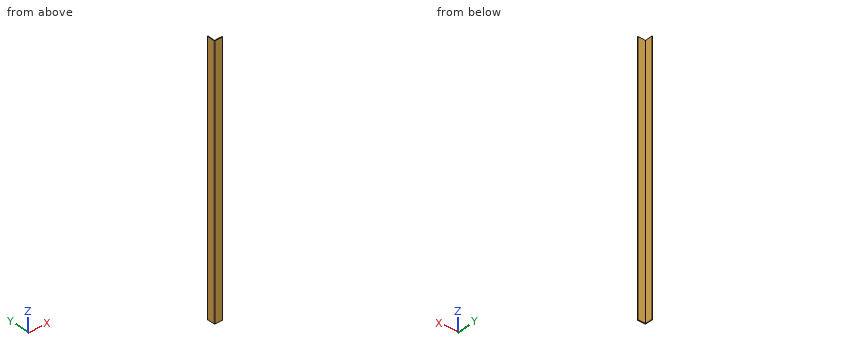
Autodesk Inventor part; units mm, degrees
ref_plane "Work Plane2" through (0, 30, 0) normal (-0.7071, 0.7071, 0) x (0, 0, -1)
ref_plane "Work Plane4" through (15.0001, 14.9999, 0) normal (-0.7071, 0.7071, 0) x (0, 0, -1)
ref_plane "YZ Plane" through (0, 0, 0) normal (1, 0, 0) x (0, 1, 0)
sketch "Sketch1" plane through (0, 0, 0) normal (0, 0, 1) x (1, 0, 0)
  line L0 (0, 0) -> (0, 30)
  line L1 (0, 0) -> (30, 0)
  line L2 (2, 30) -> (2, 2)
  line L3 (2, 2) -> (30, 2)
  line L4 (0, 30) -> (2, 30)
  line L5 (30, 2) -> (30, 0)
  dimension "d7" = 30
  dimension "d8" = 30
  dimension "d9" = 2
extrude "Extrusion1" add sketch "Sketch1" against normal blind 955
ref_plane "Work Plane1" through (2, 30, 0) normal (-0.7071, -0.7071, 0) x (0, 0, -1)
ref_plane "Work Plane2" through (0, 30, 0) normal (-0.7071, 0.7071, 0) x (0, 0, -1)
ref_plane "Work Plane3" through (30, 0, 0) normal (-0.7071, 0.7071, 0) x (0, 0, -1)
fillet "Fillet1" radius 2 1 edges at (0, 0, -477.5)
ref_plane "Work Plane4" through (15.0001, 14.9999, 0) normal (-0.7071, 0.7071, 0) x (0, 0, -1)
properties part number "Angulo en V"
Could you check a few things on this model? Use its own coordinates, in mm. Round coordinates to 2 decimals unless told otherwise and drop trailing zeros. Order: outer loops, then holes, each group sorted by start corner. A loop starts at its lowest first (then second) coordinate and runs counter-clockwise, first axis right, second up. Notation, with made-up numbers: (87.5, 84) -> (108.5, 84) arc R30 cw to (108.5, 116) -> close; hole circle Ø9 at (56.5, 24.5). An arc over 180 degrees is marked (long way). One line per question, with ' | ' between items.
Q1. If we section it at B-B on y = 17: Write out the boundary of the cut face in (x, z), plus the area to 3 significant figures.
Computed values:
outline: (0, -955) -> (2, -955) -> (2, 0) -> (0, 0) -> close | area: 1,910 mm²
Q2. If I drill on line 1 (Y direction, x = 9, z = -850.5); line 2 (X direction, y = 1.5, z = -478.5), over which ranges is the centre line in solid material (lowest first)? Write a range as from..to.
Computed values:
line 1: 0..2 | line 2: 0.06..30
Q3. If we section it at A-A on z = -384: Write out the boundary of the cut face in (x, y), plus the area to 3 significant figures.
Computed values:
outline: (0, 2) arc R2 ccw to (2, 0) -> (30, 0) -> (30, 2) -> (2, 2) -> (2, 30) -> (0, 30) -> close | area: 115 mm²
Q4. I'm going to push flat-ended pins straight in: pin 1 (8.5 mm diameter, centred on y = 13, z = -493, fed in from +X); pin 2 (12 mm diameter, centred on x = 25, z = -692.5, fed in from +Y); pin 3 (1.5 mm diameter, centred on x = 9.5, y = 3.5, fed in from -Z). Where does each tip first touch, or does it pass through?
Computed values:
pin 1: x = 2 | pin 2: y = 2 | pin 3: through
